Read the model definition and answer for the solid it produces. Units are mm, in the model's axes. Give positions to 0.01 mm unless a question says otherwise; leave off trailing zeros. Order: outer loops, then holes, each group sorted by start corner. A loop starts at its lowest first (then second) coordinate and runs counter-clockwise, first axis right, second up. Notation, with made-up numbers: (35.5, 64.25) - (65.5, 64.25) arc R15 ccw to (65.5, 80.25) - close; hole circle Ø5 at (-36.5, -27.5). An arc over 180 degrees is marked (long way). Write each question's results on one line, items separated by ' | '. Start each with the question number.
Q1. Find section C-C on x = 123.5. Give the vertices of the cut face in (y, z), and give its area (3 significant figures).
Q2. Find section B-B on x = 74. Give the vertices of the cut face in (y, z), and give its area (3 significant figures).
Q3. Find section A-A on y = 25.5. Give the vertices of the cut face in (x, z), and give its area (3 significant figures).
Q4. A flat-ended cylindrical pin translates along its axis: P1, Ø1.5, axis at y = 60, z = 1, coming from the -X side. Find the tip coordinate at first contact, or state that the pin passes through.
Q5. Find the intervals of material crossed by line 1 along X through (y, z) = (37, 0.75); line 2 along Y through (x, z) = (82, 0.2); line 3 along Y through (x, z) = (29, 1.05), in increasing order. Write a range as from..to.
from build123d import *

# Parameters (mm, degrees)
P_IDAT_VYSUNUT_M1_DEPTH = 3


with BuildPart() as part:
    # Skica1 → Přidat vysunutím1 (new body)
    with BuildSketch(Plane.XY):
        Polygon((20, 3), (35, 3), (35, 0), (55, 0), (55, 3), (70, 3), (70, 0), (77.5, 0), (77.5, 15), (52.5, 15), (52.5, 40), (77.5, 40), (77.5, 62), (70, 62), (70, 59), (55, 59), (55, 62), (35, 62), (35, 59), (20, 59), (20, 62), (0, 62), (0, 0), (20, 0), align=None)
    p_idat_vysunut_m1 = extrude(amount=P_IDAT_VYSUNUT_M1_DEPTH)

    # Zrcadlit1: Přidat vysunutím1 across plane
    add(p_idat_vysunut_m1.mirror(Plane(origin=(77.5, 0, 3), x_dir=(0, 0, 1), z_dir=(-1, 0, 0))))


solid = part.part
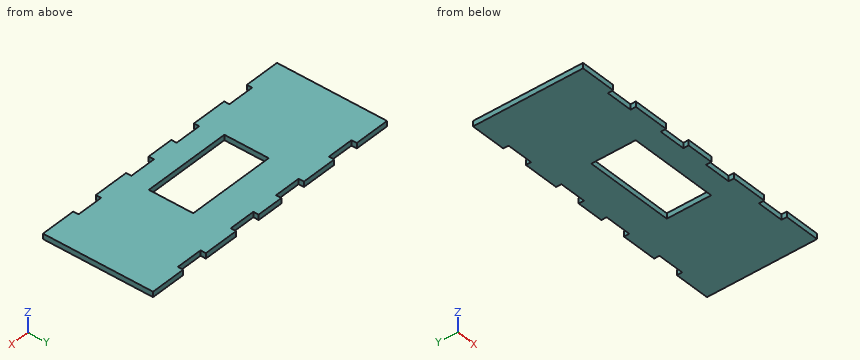
Working result:
1) outline: (3, 0) - (59, 0) - (59, 3) - (3, 3) - close | area: 168 mm²
2) outline: (0, 0) - (15, 0) - (15, 3) - (0, 3) - close; (40, 0) - (62, 0) - (62, 3) - (40, 3) - close | area: 111 mm²
3) outline: (0, 0) - (52.5, 0) - (52.5, 3) - (0, 3) - close; (102.5, 0) - (155, 0) - (155, 3) - (102.5, 3) - close | area: 315 mm²
4) P1: x = 0
5) line 1: 0..52.5, 102.5..155 | line 2: 0..15, 40..62 | line 3: 3..59
